Verification items for the finished model (mm, model axes). A direction names the side the tool comes from. Coordinates: 2 decimals unless noted, no trailing zeros. Order: outer loops, then holes, each group sorted by start corner. A loop starts at its lowest first (then second) coordinate and runs counter-clockwise, first axis right, second up. Notation, with made-up numbers: (-10, -23) -> (43, -23) arc R20 ccw to (43, 11) -> close; hole circle Ø9 at (66.25, 36). An arc over 180 degrees is marked (long way). Write item = value, one per line. Start each with the question number.
1. Cross-section at B-B on y = -6.5. Record the cut outline in (x, z).
2. Release check for a two-part mould opening along Z. For faces 1 (the flat face through (-87.75, 8.33, 48.95)), 2 (the cylindrical face through (-100.6, -28, 63.8)), 3 (the flat face through (45, -10, 5)) record: +Z half, -Z half, draft (parallel to the pull), parting line (faces both ways), or undercut.
3. Go/stop test with flat-tipped pins: P1, Ø1.5, axis at y = 21.5, z = 72, coming from the -X side; P2, Ø1, axis at x = -81.5, y = 28.5, coming from the +Z side; P3, Ø6, axis at x = -72, y = -21, coming from the +Z side. Record where each tip stops, or that it passes through.
4. Set-up check for faces 4 (the flat face through (-1, -1, 0)), 5 (the flat face through (-70.14, -9.45, 58.47)), 6 (the flat face through (45, 10, 5)): record each of +Z, -Z, +X, -X, +Y, -Y from which the full face is reachable in a straight line by a thin tool's end or side.
5. Cross-section at A-A on x = 40. Record the cut outline in (y, z), plus the area to 3 significant figures.
6. Thickness scan on line 1 along Y through (x, z) = (26.5, 8); line 2 along Z through (x, y) = (1.5, 34.5); line 3 along Z through (x, y) = (-57, 31). Record the ranges inside material, lowest first. Write a range as from..to.
7. Cross-section at D-D on x = -14.5. Record the cut outline in (y, z), plus the area to 3 significant figures.
8. Cross-section at C-C on y = 30. Record the cut outline in (x, z).
from build123d import *

# Parameters (mm, degrees)
F1_DEPTH      = 40
F1_DEPTH_BACK = 40
F2_R          = 39.99999
F4_DEPTH      = 25
F5_R          = 20
F6_R          = 5
F8_DEPTH      = 63


# Not quite as in the source:
# - a fillet or chamfer is up to 0.001 mm smaller than in the source, because OpenCascade refuses the exact size


with BuildPart() as f1:
    # F0 (on Front) → F1 (new body, two sides)
    with BuildSketch(Plane.XZ) as f1_sk:
        Polygon((-75, 0), (0, 0), (75, 0), (75, 10), (-35.3732482667, 10), (-47.8156610838, 35.5107267975), (-74.1179298912, 89.4383695755), (-83.1058703542, 85.0546581076), (-56.8036015468, 31.1270153297), (-74.7794824728, 22.3595923939), (-101.0817512801, 76.2872351718), (-110.0696917431, 71.9035237039), align=None)
    extrude(amount=F1_DEPTH)
    extrude(f1_sk.sketch, amount=-F1_DEPTH_BACK)

    # F2 (radius 40 in the source; OpenCascade refuses exactly that, so slightly less here)
    f2_edges = [f1.edges().sort_by_distance(p)[0] for p in [
        (-78.6119, -40, 87.246514),
        (-78.6119, 40, 87.246514),
        (-105.575722, -40, 74.095379),
        (-105.575722, 40, 74.095379),
    ]]
    fillet(f2_edges, radius=F2_R)

    # F3 (on face) → F4 (cut)
    with BuildSketch(Plane.XY.offset(10)):
        with BuildLine():
            Line((75, 10), (15, 10))
            ThreePointArc((15, 10), (5, 0), (15, -10))
            Line((15, -10), (75, -10))
            Line((75, -10), (75, 10))
        make_face()
    extrude(amount=-F4_DEPTH, mode=Mode.SUBTRACT)

    # F5
    f5_edges = [f1.edges().sort_by_distance(p)[0] for p in [
        (75, 40, 5),
        (75, -40, 5),
    ]]
    fillet(f5_edges, radius=F5_R)

    # F6
    f6_edges = [f1.edges().sort_by_distance(p)[0] for p in [
        (-35.373248, 0, 10),
    ]]
    fillet(f6_edges, radius=F6_R)

    # F7 (on face) → F8 (cut)
    with BuildSketch(Plane(origin=(-24.6355434727, 0, -12.0155573887), x_dir=(0, 1, 0), z_dir=(0.8987940463, 0, 0.4383711468))):
        with BuildLine():
            ThreePointArc((0, 64.3188986308), (7.0710678119, 67.247830819), (10, 74.3188986308))
            ThreePointArc((10, 74.3188986308), (-7.0710678119, 81.3899664427), (0, 64.3188986308))
        make_face()
    extrude(amount=-F8_DEPTH, mode=Mode.SUBTRACT)


solid = f1.part
Worked out:
q1.outline = (-109.84, 71.43) -> (-96.5, 44.08) -> (-87.51, 48.46) -> (-100.85, 75.81) -> close; (-89.84, 30.42) -> (-75, 0) -> (7.4, 0) -> (7.4, 10) -> (-32.25, 10) arc R5 cw to (-36.74, 12.81) -> (-53.88, 47.95) -> (-62.87, 43.57) -> (-56.8, 31.13) -> (-74.78, 22.36) -> (-80.85, 34.8) -> close; (-82.87, 84.58) -> (-69.53, 57.23) -> (-60.55, 61.61) -> (-73.88, 88.96) -> close
q2.face_1 = undercut
q2.face_2 = +Z half
q2.face_3 = draft
q3.P1 = -77.1
q3.P2 = 37.16
q3.P3 = 85.59
q4.face_4 = -Z, +X, -X, +Y, -Y
q4.face_5 = +Y, -Y
q4.face_6 = +Z, -Z, +X
q5.outline = (-40, 0) -> (-10, 0) -> (-10, 10) -> (-40, 10) -> close; (10, 0) -> (40, 0) -> (40, 10) -> (10, 10) -> close
q5.area = 600 mm²
q6.line_1 = -40..-10, 10..40
q6.line_2 = 0..10
q6.line_3 = 0..31.03, 31.53..54.34
q7.outline = (-40, 0) -> (40, 0) -> (40, 10) -> (-40, 10) -> close
q7.area = 800 mm²
q8.outline = (-104.13, 59.73) -> (-75, 0) -> (72.32, 0) -> (72.32, 10) -> (-32.25, 10) arc R5 cw to (-36.74, 12.81) -> (-68.18, 77.27) -> (-77.17, 72.88) -> (-56.8, 31.13) -> (-74.78, 22.36) -> (-95.15, 64.12) -> close
